Verification items for the finished model (mm, model axes). A direction names the side the tool comes from. Coordinates: 2 decimals unless noted, no trailing zeros. Loops run counter-clockwise (first coordinate to the right, second up) from the corner with the lowest first, then second, coordinate; pieces in that order, holes last. Notation, with made-up numbers: (-19.5, 21) - (-5.5, 21) arc R18 ccw to (-5.5, 34) - close; hole circle Ø10 at (13.5, 27.5). An arc over 180 degrees is marked (long way). One line per item, written item: value. Start each with the question number.
(1) Section check C-C (y = 79.5). Record the boundary of the cut face in (x, z).
(2) Thickness scan on probe 1 along Z at (x, y) = (92, 45.5); probe 2 along Y at (x, z) = (73.5, 24.75); probe 3 along Y at (x, z) = (8, 14.5). Record the ranges inside material, lowest first. Write a range as [from, to].
(3) Set-up check for faces 1 (the face through (65, 32, 12)), 2 (the face through (67, 52, 26)), 3 (the face through (72.17, 72.08, 12.68)): record each of +Z, -Z, +X, -X, +Y, -Y from which the full face is reachable in a straight line by a thin tool's end or side.
(4) Section check A-A (z = 13.5). Record the boundary of the cut face in (x, y).
(5) Section check B-B (x = 91). Record the boundary of the cut face in (y, z).
(6) Draft check along Y on faces 4 (the face through (0, 80, 13)), 5 (the face through (4.5, 101.9, 12.7)), 6 (the face through (101.906, 4.387, 12.675)), 7 (the face through (73.098, 72.565, 12.563)). Enter one of: +Y half, -Y half, draft (parallel to the pull), parting line (faces both ways), or undercut.
(7) Section check D-D (x = 73). Record the boundary of the cut face in (y, z), plus the area to 3 significant figures.
(8) Gauge pin test, flat ends, axial feed: P1, Ø8, axis at x = 50.5, z = 14.5, coming from the +Y side; P2, Ø12, axis at x = 57.5, z = 9.5, coming from the -Y side; P3, Ø6, axis at y = 87, z = 5.5, coming from the +X side. Record the tip position at first contact, or that the pin passes through.
```python
from build123d import *

# Parameters (mm, degrees)
CYLINDER008_W          = 102
CYLINDER008_H          = 27
CYLINDER008_ANGLE      = 5
CYLINDER007_W          = 103
CYLINDER007_H          = 27
CYLINDER007_ANGLE      = 5
CUT003_PLACEMENT_ANGLE = 85
CYLINDER004_W          = 102
CYLINDER004_H          = 27
CYLINDER004_ANGLE      = 5
CYLINDER003_W          = 103
CYLINDER003_H          = 27
CYLINDER003_ANGLE      = 5
CYLINDER005_W          = 102
CYLINDER005_H          = 27
CYLINDER005_ANGLE      = 5
CYLINDER006_W          = 103
CYLINDER006_H          = 27
CYLINDER006_ANGLE      = 5
CUT002_PLACEMENT_ANGLE = 42.5
BOX_W                  = 65
BOX_H                  = 65
BOX_DEPTH              = 27
CYLINDER001_W          = 103
CYLINDER001_H          = 1
CYLINDER001_ANGLE      = 90
CYLINDER002_W          = 103
CYLINDER002_H          = 1
CYLINDER002_ANGLE      = 90
CYLINDER_W             = 100
CYLINDER_H             = 25
CYLINDER_ANGLE         = 90


with BuildPart() as zylinder008:
    # Cylinder008 → Cylinder008 (revolve)
    with BuildSketch(Plane(origin=(0, 0, -1), x_dir=(1, 0, 0), z_dir=(0, -1, 0))):
        with Locations((51, 13.5)):
            Rectangle(CYLINDER008_W, CYLINDER008_H)
    revolve(axis=Axis((0, 0, -1), (0, 0, 1)), revolution_arc=CYLINDER008_ANGLE)


with BuildPart() as cut003:
    # Cylinder007 → Cylinder007 (revolve)
    with BuildSketch(Plane(origin=(0, 0, -1), x_dir=(1, 0, 0), z_dir=(0, -1, 0))):
        with Locations((51.5, 13.5)):
            Rectangle(CYLINDER007_W, CYLINDER007_H)
    revolve(axis=Axis((0, 0, -1), (0, 0, 1)), revolution_arc=CYLINDER007_ANGLE)

    # Cut003: cut Zylinder008
    add(zylinder008.part, mode=Mode.SUBTRACT)


with BuildPart() as cut003_1:
    # Cut003 placement: moved
    add(cut003.part.rotate(Axis((0, 0, 0), (0, 0, 1)), CUT003_PLACEMENT_ANGLE))


with BuildPart() as zylinder004:
    # Cylinder004 → Cylinder004 (revolve)
    with BuildSketch(Plane(origin=(0, 0, -1), x_dir=(1, 0, 0), z_dir=(0, -1, 0))):
        with Locations((51, 13.5)):
            Rectangle(CYLINDER004_W, CYLINDER004_H)
    revolve(axis=Axis((0, 0, -1), (0, 0, 1)), revolution_arc=CYLINDER004_ANGLE)


with BuildPart() as cut001:
    # Cylinder003 → Cylinder003 (revolve)
    with BuildSketch(Plane(origin=(0, 0, -1), x_dir=(1, 0, 0), z_dir=(0, -1, 0))):
        with Locations((51.5, 13.5)):
            Rectangle(CYLINDER003_W, CYLINDER003_H)
    revolve(axis=Axis((0, 0, -1), (0, 0, 1)), revolution_arc=CYLINDER003_ANGLE)

    # Cut001: cut Zylinder004
    add(zylinder004.part, mode=Mode.SUBTRACT)


with BuildPart() as zylinder005:
    # Cylinder005 → Cylinder005 (revolve)
    with BuildSketch(Plane(origin=(0, 0, -1), x_dir=(1, 0, 0), z_dir=(0, -1, 0))):
        with Locations((51, 13.5)):
            Rectangle(CYLINDER005_W, CYLINDER005_H)
    revolve(axis=Axis((0, 0, -1), (0, 0, 1)), revolution_arc=CYLINDER005_ANGLE)


with BuildPart() as cut002:
    # Cylinder006 → Cylinder006 (revolve)
    with BuildSketch(Plane(origin=(0, 0, -1), x_dir=(1, 0, 0), z_dir=(0, -1, 0))):
        with Locations((51.5, 13.5)):
            Rectangle(CYLINDER006_W, CYLINDER006_H)
    revolve(axis=Axis((0, 0, -1), (0, 0, 1)), revolution_arc=CYLINDER006_ANGLE)

    # Cut002: cut Zylinder005
    add(zylinder005.part, mode=Mode.SUBTRACT)


with BuildPart() as cut002_1:
    # Cut002 placement: moved
    add(cut002.part.rotate(Axis((0, 0, 0), (0, 0, 1)), CUT002_PLACEMENT_ANGLE))


with BuildPart() as obj1:
    # Box → Box (new body)
    with BuildSketch(Plane.XY.offset(-1)):
        with Locations((32.5, 32.5)):
            Rectangle(BOX_W, BOX_H)
    extrude(amount=BOX_DEPTH)


with BuildPart() as zylinder001:
    # Cylinder001 → Cylinder001 (revolve)
    with BuildSketch(Plane(origin=(0, 0, -1), x_dir=(1, 0, 0), z_dir=(0, -1, 0))):
        with Locations((51.5, 0.5)):
            Rectangle(CYLINDER001_W, CYLINDER001_H)
    revolve(axis=Axis((0, 0, -1), (0, 0, 1)), revolution_arc=CYLINDER001_ANGLE)


with BuildPart() as zylinder002:
    # Cylinder002 → Cylinder002 (revolve)
    with BuildSketch(Plane(origin=(0, 0, 25), x_dir=(1, 0, 0), z_dir=(0, -1, 0))):
        with Locations((51.5, 0.5)):
            Rectangle(CYLINDER002_W, CYLINDER002_H)
    revolve(axis=Axis((0, 0, 25), (0, 0, 1)), revolution_arc=CYLINDER002_ANGLE)


with BuildPart() as fusion001:
    # Cylinder → Cylinder (revolve)
    with BuildSketch(Plane.XZ):
        with Locations((50, 12.5)):
            Rectangle(CYLINDER_W, CYLINDER_H)
    revolve(axis=Axis((0, 0, 0), (0, 0, 1)), revolution_arc=CYLINDER_ANGLE)

    # Fusion: union Zylinder001, Zylinder002
    add(zylinder001.part)
    add(zylinder002.part)

    # Cut: cut obj1
    add(obj1.part, mode=Mode.SUBTRACT)

    # Fusion001: union Cut003, Cut001, Cut002
    add(cut003_1.part)
    add(cut001.part)
    add(cut002_1.part)


solid = fusion001.part
```
Responses:
1. outline: (0, -1) - (65.49, -1) - (65.49, 0) - (60.66, 0) - (60.66, 25) - (65.49, 25) - (65.49, 26) - (0, 26) - close
2. probe 1: z = [-1, 0], [25, 26]
2. probe 2: y = [0, 67.81], [70.72, 72.16]
2. probe 3: y = [65, 99.68], [101.69, 102.69]
3. face 1: +Z, -Z, -X, -Y
3. face 2: +Z, +X, -X, +Y, -Y
3. face 3: none
4. outline: (0, 65) - (65, 65) - (65, 0) - (100, 0) arc R100 ccw to (0, 100) - close; (0, 102) arc R102 cw to (8.89, 101.61) - (8.98, 102.61) arc R103 ccw to (0, 103) - close; (68.91, 75.2) arc R102 cw to (75.2, 68.91) - (75.94, 69.59) arc R103 ccw to (69.59, 75.94) - close; (101.61, 8.89) arc R102 cw to (102, 0) - (103, 0) arc R103 ccw to (102.61, 8.98) - close
5. outline: (0, -1) - (48.25, -1) - (48.25, 0) - (41.46, 0) - (41.46, 25) - (48.25, 25) - (48.25, 26) - (0, 26) - close
6. face 4: draft
6. face 5: undercut
6. face 6: -Y half
6. face 7: +Y half
7. outline: (0, -1) - (72.66, -1) - (72.66, 26) - (0, 26) - close; hole (68.34, 0) - (71.24, 0) - (71.24, 25) - (68.34, 25) - close
7. area: 1,890 mm²
8. P1: stops at y = 88.53
8. P2: stops at y = 65
8. P3: stops at x = 54.26
